from build123d import *

# Parameters (mm, degrees)
CROQUIS1_W                         = 60
CROQUIS1_H                         = 38
SALIENTE_EXTRUIR1_DEPTH            = 22
CROQUIS2_R                         = 5.1
CORTAR_EXTRUIR1_DEPTH              = 61
TALADROS_DE_ESPIGA_DE_4_0MM2_D     = 4
TALADROS_DE_ESPIGA_DE_4_0MM2_DEPTH = 14
TALADROS_DE_ESPIGA_DE_4_0MM2_TIP   = 1.201721238
CROQUIS6_W                         = 60
CROQUIS6_H                         = 3
SALIENTE_EXTRUIR2_DEPTH            = 3
TALADRO_ROSCADO_M31_D              = 2.5
TALADRO_ROSCADO_M31_DEPTH          = 14
TALADRO_ROSCADO_M31_TIP            = 0.751075774
TALADRO_DE_MARGEN_PARA_M41_D       = 4.5


with BuildPart() as part:
    # Croquis1 → Saliente-Extruir1 (new body)
    with BuildSketch(Plane.XY):
        with Locations((30, 19)):
            Rectangle(CROQUIS1_W, CROQUIS1_H)
    extrude(amount=SALIENTE_EXTRUIR1_DEPTH)

    # Croquis2 → Cortar-Extruir1 (cut, through all)
    with BuildSketch(Plane(origin=(60, 0, 0), x_dir=(0, 0, -1), z_dir=(1, 0, 0))):
        with Locations((-7.5, 20.5)):
            Circle(CROQUIS2_R)
    extrude(amount=-CORTAR_EXTRUIR1_DEPTH, mode=Mode.SUBTRACT)

    # Taladros de espiga de Ø4.0mm2
    with Locations(Plane.XY.offset(22)):
        with Locations((30, 6), (30, 32)):
            Hole(TALADROS_DE_ESPIGA_DE_4_0MM2_D / 2, depth=TALADROS_DE_ESPIGA_DE_4_0MM2_DEPTH)
            with Locations((0, 0, -(TALADROS_DE_ESPIGA_DE_4_0MM2_DEPTH + TALADROS_DE_ESPIGA_DE_4_0MM2_TIP / 2))):  # 118° drill point
                Cone(0, TALADROS_DE_ESPIGA_DE_4_0MM2_D / 2, TALADROS_DE_ESPIGA_DE_4_0MM2_TIP, mode=Mode.SUBTRACT)

    # Croquis6 → Saliente-Extruir2 (add)
    with BuildSketch(Plane(origin=(0, 0, 0), x_dir=(-1, 0, 0), z_dir=(0, 0, -1))):
        with Locations((-30, 36.5)):
            Rectangle(CROQUIS6_W, CROQUIS6_H)
    extrude(amount=SALIENTE_EXTRUIR2_DEPTH)

    # Taladro roscado M31
    with Locations(Plane(origin=(60, 0, 0), x_dir=(0, 0, -1), z_dir=(1, 0, 0))):
        with Locations((-15.5, 20.5), (-7.5, 12.5), (-7.5, 28.5)):
            Hole(TALADRO_ROSCADO_M31_D / 2, depth=TALADRO_ROSCADO_M31_DEPTH)
            with Locations((0, 0, -(TALADRO_ROSCADO_M31_DEPTH + TALADRO_ROSCADO_M31_TIP / 2))):  # 118° drill point
                Cone(0, TALADRO_ROSCADO_M31_D / 2, TALADRO_ROSCADO_M31_TIP, mode=Mode.SUBTRACT)

    # Taladro de margen para M41 (through all)
    with Locations(Plane.XY.offset(22)):
        with Locations((43, 5), (43, 31), (17, 5), (17, 31)):
            Hole(TALADRO_DE_MARGEN_PARA_M41_D / 2)


solid = part.part
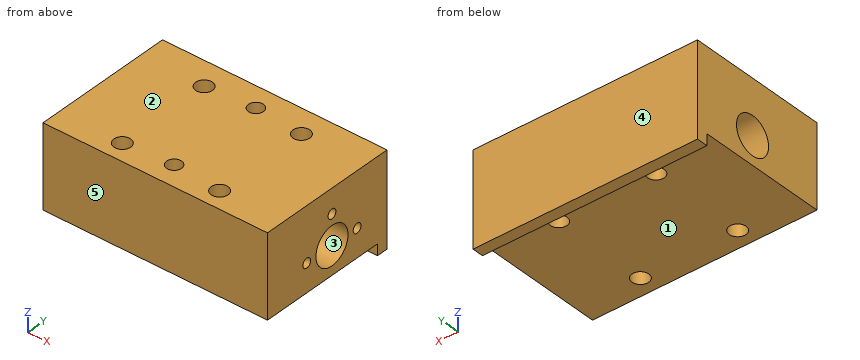
Part model, mm, in its own coordinate system. Face numbers are marked on the shaded views. A direction names the side the tool comes from. Coordinates: 2 decimals unless noted, no trailing zeros. Loops run counter-clockwise (first coordinate to the right, second up) from the corner with the lowest first, then second, coordinate; pieces in that order, holes last. Notation, with made-up numbers: (48.5, 23) - (89.5, 23) arc R9 cw to (89.5, 39) - close; hole circle Ø3 at (56.5, 57.25). An arc over 180 degrees is marked (long way). Write each question's results on one line, items separated by ' | '. Start each with the question number.
Q1. Probe line 1 along Y through (x, z) = (52, 15.5); line 2 along Z through (x, y) = (50.25, 12.5); line 3 along X through (y, z) = (32, 14.75). List the from-to ranges inside material, lowest first.
Q2. Two-plate mould, pull along Y, no slides. Class the marked faces 3, 4 and 5: +Y half, -Y half, draft (parallel to the pull), parting line (faces both ways), or undercut.
Q3. Slice it at C-C on y = 24.5. Give the cut face in (x, z).
Q4. Slice it at A-A on x = 17. Give the cut face in (y, z), and give its area (3 significant figures).
Q5. Which spindle directions (+Z, -Z, +X, -X, +Y, -Y) get a long thin tool onto all of the face, cutting with end or side? Do the marked faces 1 and 2. Say none if no direction does.
Q6. Slice it at D-D on x = 47. Give the cut face in (y, z), and give its area (3 significant figures).
Q7. Drop flat-ended pins along their axis: pin 1 Ø6 at (x, y) = (43, 5) entering from +Z; pin 2 Ø1.5 at (x, z) = (39, -2) entering from -Y; pin 3 Ø1 at (x, y) = (45.5, 4.5) entering from -Z; pin 4 Ø2 at (y, z) = (12.5, 7.5) entering from +X. Give the stop position or say it passes through.
Q8. Slice it at B-B on x = 26.5. Give the cut face in (y, z), and give its area (3 significant figures).
Answer:
1) line 1: y = 0 to 19.25, 21.75 to 38 | line 2: z = 0 to 6.25, 8.75 to 22 | line 3: x = 0 to 14.98, 19.02 to 28, 32 to 40.98, 45.02 to 60
2) face 3: undercut | face 4: +Y half | face 5: -Y half
3) outline: (0, 0) - (60, 0) - (60, 4.34) - (0, 4.34) - close; (0, 10.66) - (60, 10.66) - (60, 22) - (0, 22) - close
4) outline: (0, 0) - (2.75, 0) - (2.75, 22) - (0, 22) - close; (7.25, 0) - (28.75, 0) - (28.75, 22) - (7.25, 22) - close; (33.25, 0) - (35, 0) - (35, -3) - (38, -3) - (38, 22) - (33.25, 22) - close; hole circle Ø10.2 at (20.5, 7.5) | area: 565 mm2
5) face 1: -Z, +X, -X, -Y | face 2: +Z, +X, -X, +Y, -Y
6) outline: (0, 0) - (35, 0) - (35, -3) - (38, -3) - (38, 22) - (0, 22) - close; hole circle Ø2.5 at (12.5, 7.5); hole circle Ø10.2 at (20.5, 7.5); hole circle Ø2.5 at (20.5, 15.5); hole circle Ø2.5 at (28.5, 7.5) | area: 749 mm2
7) pin 1: stops at z = 22 | pin 2: stops at y = 35 | pin 3: stops at z = 0 | pin 4: stops at x = 45.85
8) outline: (0, 0) - (35, 0) - (35, -3) - (38, -3) - (38, 22) - (0, 22) - close; hole circle Ø10.2 at (20.5, 7.5) | area: 763 mm2
